Work out the finished part from the listing and answer in its coordinate system (mm). A direction names the side the tool comes from. Coordinates: 2 decimals unless noted, no trailing zeros. Order: outer loops, then holes, each group sorted by start corner. A loop starts at its lowest first (then second) coordinate and runs counter-clockwise, first axis right, second up. Notation, with made-up numbers: M 44.5,70 L 53.5,70 A25 cw 53.5,92 Z; hole C -7.5,-10.75 d10. An arc over 180 degrees is marked long. Use a Markdown table: item, result.
from build123d import *

# Parameters (mm, degrees)
PAD013_DEPTH    = 19
FILLET001_R     = 20
SKETCH022_R     = 2
POCKET013_DEPTH = 19.001
SKETCH027_R     = 2
POCKET017_DEPTH = 19.001
SKETCH069_R     = 2
POCKET044_DEPTH = 19.001


with BuildPart() as part:
    # Sketch015 → Pad013 (new body)
    with BuildSketch(Plane.XY):
        with BuildLine():
            Line((-275, 216.2), (-238, 216.2))
            Line((-238, 216.2), (-238, 25))
            ThreePointArc((-238, 25), (-263, 0), (-238, -25))
            Line((-238, -25), (-238, -35))
            Line((-238, -35), (-151.2, -121.8))
            Line((-151.2, -121.8), (-41.2, -121.8))
            Line((-41.2, -121.8), (18.8, -61.8))
            Line((159.572483, -61.8), (18.8, -61.8))
            ThreePointArc((159.572483, -61.8), (202.10651, -87.039578), (251.554314, -85.993421))
            Line((251.554314, -85.993421), (275, -126.60254))
            Line((275, -126.60254), (275, -133.8))
            Line((275, -133.8), (-275, -133.8))
            Line((-275, -133.8), (-275, 216.2))
        make_face()
    extrude(amount=PAD013_DEPTH)

    # Fillet001
    fillet001_edges = [part.edges().sort_by_distance(p)[0] for p in [
        (-275, 216.2, 9.5),
        (-275, -133.8, 9.5),
    ]]
    fillet(fillet001_edges, radius=FILLET001_R)

    # Sketch022 (on Face5 of Fillet001) → Pocket013 (cut, through all)
    with BuildSketch(Plane.XY.offset(19)):
        with Locations((-255, 196.2)):
            Circle(SKETCH022_R)
        with Locations((-255, -113.8)):
            Circle(SKETCH022_R)
        with Locations((215, -113.8)):
            Circle(SKETCH022_R)
    extrude(amount=-POCKET013_DEPTH, mode=Mode.SUBTRACT)

    # Sketch027 (on Face5 of Pocket013) → Pocket017 (cut, through all)
    with BuildSketch(Plane.XY.offset(19)):
        with Locations((255, -113.8)):
            Circle(SKETCH027_R)
    extrude(amount=-POCKET017_DEPTH, mode=Mode.SUBTRACT)

    # Sketch069 (on Face5 of Pocket017) → Pocket044 (cut, through all)
    with BuildSketch(Plane.XY.offset(19)):
        with Locations((-217.5, -77)):
            Circle(SKETCH069_R)
        with Locations((-217.5, -121)):
            Circle(SKETCH069_R)
    extrude(amount=-POCKET044_DEPTH, mode=Mode.SUBTRACT)


with BuildPart() as part_1:
    # Body009 placement: moved
    add(part.part.moved(Location((0, 0, -9))))


solid = part_1.part
(1) Which of the six approach directions +Z, -Z, +X, -X, +Y, -Y give full straight-line access (tool end or side, diameter ignored) to faces 5 (the flat face through (-238, 122, 0)), 6 (the flat face through (-11.6, -92.2, 0.4)), 7 (the cylindrical face through (-268.986, 210.497, 0.633))?
Conclusion:
| item | result |
|---|---|
| face 5 | +Z, -Z, +X, +Y |
| face 6 | +Z, -Z, +Y |
| face 7 | +Z, -Z, -X, +Y |
(2) A cutting plane is placed at B-B (x = -29). Determine the outline of the cut face in (y, z), then the cut area to 3 significant figures.
Conclusion:
| item | result |
|---|---|
| outline | M -133.8,-9 L -109.6,-9 L -109.6,10 L -133.8,10 Z |
| area | 460 mm2 |
(3) A cutting plane is placed at A-A (z = -3.5). Determine the outline of the cut face in (x, y), then the cut area to 3 significant figures.
Conclusion:
| item | result |
|---|---|
| outline | M -275,-113.8 A20 ccw -255,-133.8 L 275,-133.8 L 275,-126.6 L 251.55,-85.99 A90 cw 159.57,-61.8 L 18.8,-61.8 L -41.2,-121.8 L -151.2,-121.8 L -238,-35 L -238,-25 A25 cw -238,25 L -238,216.2 L -255,216.2 A20 ccw -275,196.2 Z; hole C -255,-113.8 d4; hole C -255,196.2 d4; hole C -217.5,-121 d4; hole C -217.5,-77 d4; hole C 215,-113.8 d4; hole C 255,-113.8 d4 |
| area | 35,800 mm2 |
(4) Determine the mould class of faces 1 (the flat face through (263.11, -106.01, 0.37)), 2 (the flat face through (-97, -121.8, 0)), 3 (the flat face through (-195, -78, 0)), 4 (the flat face through (-275, 39, 0)) for opening direction X: pulls with the +X half, pulls with the -X half, needs draft (parallel to the pull), parting line crosses it, or undercut.
Conclusion:
| item | result |
|---|---|
| face 1 | pulls with the +X half |
| face 2 | undercut |
| face 3 | undercut |
| face 4 | pulls with the -X half |
(5) Straight lines are drawn through the part: L1, parallel to X at y = 196.2, z = -1.25; L2, parallel to Y at x = -217.5, z = 1.25; L3, parallel to Y at x = 90, z = -2. For each, find the intervals that lie inside material, in ascending order.
Conclusion:
| item | result |
|---|---|
| L1 | -275 to -257, -253 to -238 |
| L2 | -133.8 to -123, -119 to -79, -75 to -55.5 |
| L3 | -133.8 to -61.8 |
(6) Given P1, Ø4, axis at y = 75.5, z = 4.5, coming from the +X side; P2, Ø5.5, axis at x = -123, z = 0, coming from the +Y side; P3, Ø5, axis at x = 190.5, z = 2, coming from the +Y side; P4, Ø3.5, axis at x = 215, y = -113.8, coming from the +Z side, each flat-ended and moving along its own axis, determine where each tip first touches the part or whether it passes through.
Conclusion:
| item | result |
|---|---|
| P1 | x = -238 |
| P2 | y = -121.8 |
| P3 | y = -82.04 |
| P4 | through |
(7) A cutting plane is placed at C-C (y = 0). Determine the outline of the cut face in (x, z), then the cut area to 3 significant figures.
Conclusion:
| item | result |
|---|---|
| outline | M -275,-9 L -263,-9 L -263,10 L -275,10 Z |
| area | 228 mm2 |
